Part model, mm, in its own coordinate system. Face numbers are marked on the shaded views. Give positions to 0.01 mm unless a question says otherwise; leave off trailing zeros. Order: outer loops, then holes, each group sorted by start corner. A loop starts at its lowest first (then second) coordinate and runs counter-clockwise, first axis right, second up.
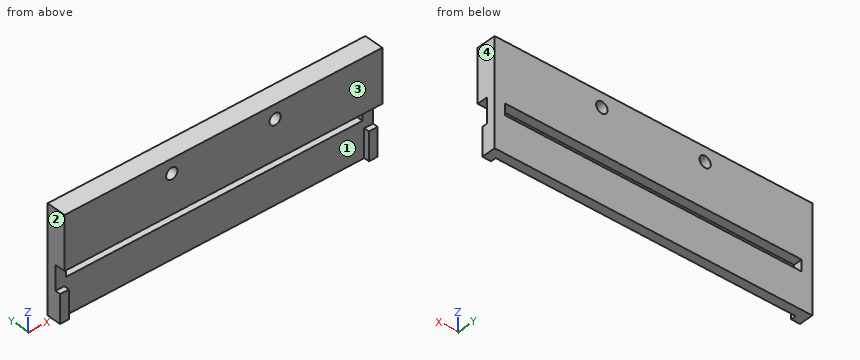
from build123d import *

# Parameters (mm, degrees)
SKETCH2_W           = 90
SKETCH2_H           = 30
BOSS_EXTRUDE1_DEPTH = 5.5
SKETCH3_W           = 90
SKETCH3_H           = 3
CUT_EXTRUDE1_DEPTH  = 1.5
SKETCH4_W           = 85
SKETCH4_H           = 1.5
CUT_EXTRUDE2_DEPTH  = 15
SKETCH5_W           = 84
SKETCH5_H           = 3.2
CUT_EXTRUDE3_DEPTH  = 2.5
SKETCH6_R           = 1.6
CUT_EXTRUDE4_DEPTH  = 48.75196331
SKETCH7_W           = 90
SKETCH7_H           = 1.5
CUT_EXTRUDE5_DEPTH  = 5
SKETCH8_W           = 90
SKETCH8_H           = 7
CUT_EXTRUDE6_DEPTH  = 3


with BuildPart() as part:
    # Sketch2 → Boss-Extrude1 (new body)
    with BuildSketch(Plane(origin=(0, 0, 0), x_dir=(1, 0, 0), z_dir=(0, 1, 0))):
        Rectangle(SKETCH2_W, SKETCH2_H)
    extrude(amount=BOSS_EXTRUDE1_DEPTH)

    # Sketch3 → Cut-Extrude1 (cut)
    with BuildSketch(Plane.XZ):
        with Locations((0, -8.5)):
            Rectangle(SKETCH3_W, SKETCH3_H)
    extrude(amount=-CUT_EXTRUDE1_DEPTH, mode=Mode.SUBTRACT)

    # Sketch4 → Cut-Extrude2 (cut)
    with BuildSketch(Plane(origin=(0, 0, -15), x_dir=(-1, 0, 0), z_dir=(0, 0, -1))):
        with Locations((0, 2.25)):
            Rectangle(SKETCH4_W, SKETCH4_H)
    extrude(amount=-CUT_EXTRUDE2_DEPTH, mode=Mode.SUBTRACT)

    # Sketch5 → Cut-Extrude3 (cut)
    with BuildSketch(Plane(origin=(0, 5.5, 0), x_dir=(1, 0, 0), z_dir=(0, 1, 0))):
        with Locations((0, 3.15)):
            Rectangle(SKETCH5_W, SKETCH5_H)
    extrude(amount=-CUT_EXTRUDE3_DEPTH, mode=Mode.SUBTRACT)

    # Sketch6 → Cut-Extrude4 (cut, through all)
    with BuildSketch(Plane(origin=(0, 5.5, 0), x_dir=(1, 0, 0), z_dir=(0, 1, 0))):
        with Locations(Location((-14.633, -11, 0), (0, 0, 270))):
            Circle(SKETCH6_R)
        with Locations(Location((14.633, -11, 0), (0, 0, 270))):
            Circle(SKETCH6_R)
    extrude(amount=-CUT_EXTRUDE4_DEPTH, mode=Mode.SUBTRACT)

    # Sketch7 → Cut-Extrude5 (cut)
    with BuildSketch(Plane(origin=(0, 0, -15), x_dir=(-1, 0, 0), z_dir=(0, 0, -1))):
        with Locations((0, 0.75)):
            Rectangle(SKETCH7_W, SKETCH7_H)
    extrude(amount=-CUT_EXTRUDE5_DEPTH, mode=Mode.SUBTRACT)

    # Sketch8 → Cut-Extrude6 (cut)
    with BuildSketch(Plane(origin=(0, 0, 0), x_dir=(-1, 0, 0), z_dir=(0, -1, 0))):
        with Locations((0, 3.5)):
            Rectangle(SKETCH8_W, SKETCH8_H)
    extrude(amount=-CUT_EXTRUDE6_DEPTH, mode=Mode.SUBTRACT)


solid = part.part
Item 1: Drop flat-ended pins along their axis: P1, Ø12, axis at x = 3.5, z = -4.5, coming from the +Y side; P2, Ø3, axis at x = -44, z = -9, coming from the -Y side; P3, Ø3, axis at x = 14.633, z = 11, coming from the -Y side; P4, Ø0.9, axis at x = -8, y = 1.5, coming from the -Z side. Give the stop position or say it passes through.
Item 2: Pull direction X, two halves, no side cores. Call the marked faces 1, 2, 3 and 4: released by +X, released by -X, zero draft, split by the parting line, or undercut.
Item 3: Band-saw the part on C-C on z = -9.5. List the corners of the cut face in (x, y), plus the area to 4 significant figures.
Item 4: Drill centre lines: probe 1 along X at (y, z) = (1.25, 11); probe 2 along Z at (x, y) = (2, 3.45); probe 3 along X at (y, z) = (2, 12.25). Where is each one in solid material? Low to high.
Item 5: Band-saw the part on A-A on z = 11. List the corners of the cut face in (x, y).
Item 6: Band-saw the part on B-B on x = 20.5. List the corners of the cut face in (y, z), plus the area to 3 significant figures.
Working result:
1. P1: stops at y = 5.5
1. P2: stops at y = 1.5
1. P3: passes through
1. P4: stops at z = 0
2. face 1: undercut
2. face 2: released by -X
2. face 3: zero draft
2. face 4: released by +X
3. outline: (-45, 1.5) - (-42.5, 1.5) - (-42.5, 3) - (42.5, 3) - (42.5, 1.5) - (45, 1.5) - (45, 5.5) - (-45, 5.5) - close
3. area: 232.5 mm2
4. probe 1: x = -45 to -16.23, -13.03 to 13.03, 16.23 to 45
4. probe 2: z = -15 to -4.75, -1.55 to 15
4. probe 3: x = -45 to -15.63, -13.63 to 13.63, 15.63 to 45
5. outline: (-45, 0) - (-16.23, 0) - (-16.23, 5.5) - (-45, 5.5) - close; (-13.03, 0) - (13.03, 0) - (13.03, 5.5) - (-13.03, 5.5) - close; (16.23, 0) - (45, 0) - (45, 5.5) - (16.23, 5.5) - close
6. outline: (0, 0) - (3, 0) - (3, -1.55) - (5.5, -1.55) - (5.5, 15) - (0, 15) - close; (3, -15) - (5.5, -15) - (5.5, -4.75) - (3, -4.75) - close
6. area: 112 mm2
